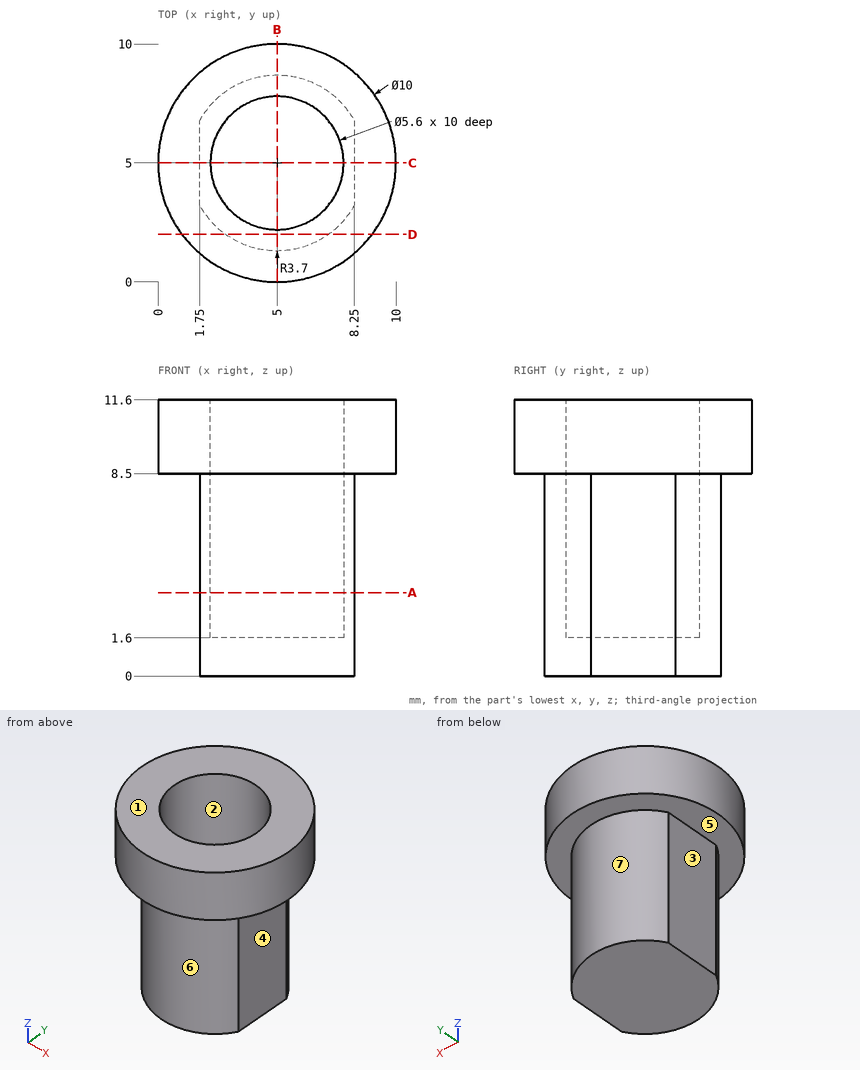
Check sheet for the drawn part. Datum: minimum x, y, z corner. Units: mm. A direction names the side the tool comes from. Round coordinates to 2 decimals unless told otherwise and drop trailing zeros. Write each loop counter-clockwise with the first axis right and the second up, starting at its lowest first coordinate (ties: lowest second). Pieces come first, ordered by that corner, then holes. Notation, with made-up numbers: (35, 15.5) -> (71, 15.5) arc R13 ccw to (71, 26.5) -> close; hole circle Ø11 at (12.25, 43). An arc over 180 degrees is marked (long way). Put each result on its own line as item: value.
(1) Sectioned sample at D-D (y = 2). Enter the section's corners in (x, z).
Values found:
outline: (1, 8.5) -> (2.83, 8.5) -> (2.83, 0) -> (7.17, 0) -> (7.17, 8.5) -> (9, 8.5) -> (9, 11.6) -> (1, 11.6) -> close
(2) Sectioned sample at A-A (z = 3.5). Enter the section's corners in (x, y).
Values found:
outline: (1.75, 3.23) arc R3.7 ccw to (8.25, 3.23) -> (8.25, 6.77) arc R3.7 ccw to (1.75, 6.77) -> close; hole circle Ø5.6 at (5, 5)
(3) Tool access check on the marked faces 4, 5, 6 and 7. Record the directions out of +Z, -Z, +X, -X, +Y, -Y that give a thin tool (end or side, any length) a straight path to the whole face; none if there is none.
Values found:
face 4: -Z, +X, +Y, -Y
face 5: -Z
face 6: -Z, -Y
face 7: -Z, +Y
(4) Sectioned sample at C-C (y = 5). Enter the section's corners in (x, z), plus the area to 4 significant figures.
Values found:
outline: (0, 8.5) -> (1.75, 8.5) -> (1.75, 0) -> (8.25, 0) -> (8.25, 8.5) -> (10, 8.5) -> (10, 11.6) -> (7.8, 11.6) -> (7.8, 1.6) -> (2.2, 1.6) -> (2.2, 11.6) -> (0, 11.6) -> close
area: 30.25 mm^2
(5) Material ranges on line 1 (Z direction, x = 4.75, y = 4.25); line 2 (Z direction, x = 7.75, y = 7.75); line 3 (X direction, y = 4.25, z = 8.75), recorded low to high.
Values found:
line 1: z = 0 to 1.6
line 2: z = 8.5 to 11.6
line 3: x = 0.06 to 2.3, 7.7 to 9.94
(6) Mould release check, pull along X, two halves, no side actions. Record for the marked faces 1, 2 and 3: released by +X, released by -X, zero draft, split by the parting line, or undercut.
Values found:
face 1: zero draft
face 2: undercut
face 3: released by -X
(7) Sectioned sample at B-B (x = 5). Enter the section's corners in (y, z).
Values found:
outline: (0, 8.5) -> (1.3, 8.5) -> (1.3, 0) -> (8.7, 0) -> (8.7, 8.5) -> (10, 8.5) -> (10, 11.6) -> (7.8, 11.6) -> (7.8, 1.6) -> (2.2, 1.6) -> (2.2, 11.6) -> (0, 11.6) -> close
(8) Go/stop test with flat-tipped pins: pin 1 Ø1.8 at (y, z) = (4.5, 3) entering from +X; pin 2 Ø2 at (x, z) = (6.5, 6.5) entering from -Y; pin 3 Ø4 at (y, z) = (4.5, 6) entering from -X. Record where each tip stops, or that it passes through.
Values found:
pin 1: stops at x = 8.25
pin 2: stops at y = 1.33
pin 3: stops at x = 1.75
